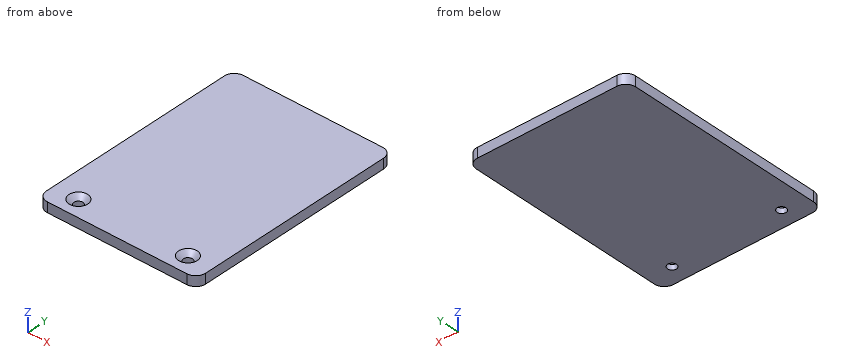
from build123d import *

# Parameters (mm, degrees)
SKETCH1_W                                           = 80
SKETCH1_H                                           = 110
BOSS_EXTRUDE1_DEPTH                                 = 5
FILLET1_R                                           = 5
CSK_FOR_M4_COUNTERSUNK_FLAT_HEAD_SCREW1_D           = 4.5
CSK_FOR_M4_COUNTERSUNK_FLAT_HEAD_SCREW1_DEPTH       = 10
CSK_FOR_M4_COUNTERSUNK_FLAT_HEAD_SCREW1_CSINK_D     = 9.4
CSK_FOR_M4_COUNTERSUNK_FLAT_HEAD_SCREW1_CSINK_ANGLE = 90
CSK_FOR_M4_COUNTERSUNK_FLAT_HEAD_SCREW1_TIP         = 1.351936393


with BuildPart() as part:
    # Sketch1 → Boss-Extrude1 (new body)
    with BuildSketch(Plane.XY):
        with Locations((0, 55)):
            Rectangle(SKETCH1_W, SKETCH1_H)
    extrude(amount=BOSS_EXTRUDE1_DEPTH)

    # Fillet1
    fillet1_edges = [part.edges().sort_by_distance(p)[0] for p in [
        (-40, 110, 2.5),
        (40, 110, 2.5),
        (40, 0, 2.5),
        (-40, 0, 2.5),
    ]]
    fillet(fillet1_edges, radius=FILLET1_R)

    # CSK for M4 Countersunk Flat Head Screw1
    with Locations(Plane.XY.offset(5)):
        with Locations((-27.5, 9), (27.5, 8.987365755)):
            CounterSinkHole(CSK_FOR_M4_COUNTERSUNK_FLAT_HEAD_SCREW1_D / 2, CSK_FOR_M4_COUNTERSUNK_FLAT_HEAD_SCREW1_CSINK_D / 2, depth=CSK_FOR_M4_COUNTERSUNK_FLAT_HEAD_SCREW1_DEPTH, counter_sink_angle=CSK_FOR_M4_COUNTERSUNK_FLAT_HEAD_SCREW1_CSINK_ANGLE)
            with Locations((0, 0, -(CSK_FOR_M4_COUNTERSUNK_FLAT_HEAD_SCREW1_DEPTH + CSK_FOR_M4_COUNTERSUNK_FLAT_HEAD_SCREW1_TIP / 2))):  # 118° drill point
                Cone(0, CSK_FOR_M4_COUNTERSUNK_FLAT_HEAD_SCREW1_D / 2, CSK_FOR_M4_COUNTERSUNK_FLAT_HEAD_SCREW1_TIP, mode=Mode.SUBTRACT)


solid = part.part
The model under review builds one solid part; all positions refer to its coordinate system, in mm. Give positions to 0.01 mm unless a question says otherwise; leave off trailing zeros. Loops run counter-clockwise (first coordinate to the right, second up) from the corner with the lowest first, then second, coordinate; pieces in that order, holes last. Notation, with made-up numbers: (-7.5, 1.25) -> (50.5, 1.25) arc R19 ccw to (50.5, 24.25) -> close; hole circle Ø8 at (43, 16). An arc over 180 degrees is marked (long way). Put each result on its own line as item: value. Start each with the question number.
1. Wall thickness on probe 1 along Y at (x, z) = (-27.5, 1.8); probe 2 along X at (y, z) = (9, 0.7); probe 3 along Y at (x, z) = (27.5, 1.7): over which ranges is each line inside the solid? List them lowest first.
2. Clearance check with a flat-ended pin moving along its axis: P1, Ø7, axis at x = -27.5, y = 9, coming from the +Z side. State where the tip first meets the part, or that it passes through.
3. We need section A-A on x = -27.5. State the section outline as (y, z) points, then the cut area to 3 significant figures.
Determined:
1. probe 1: 0 to 6.75, 11.25 to 110
1. probe 2: -40 to -29.75, -25.25 to 25.25, 29.75 to 40
1. probe 3: 0 to 6.74, 11.24 to 110
2. P1: z = 3.8
3. outline: (0, 0) -> (6.75, 0) -> (6.75, 2.55) -> (4.3, 5) -> (0, 5) -> close; (11.25, 0) -> (110, 0) -> (110, 5) -> (13.7, 5) -> (11.25, 2.55) -> close
3. area: 521 mm^2
